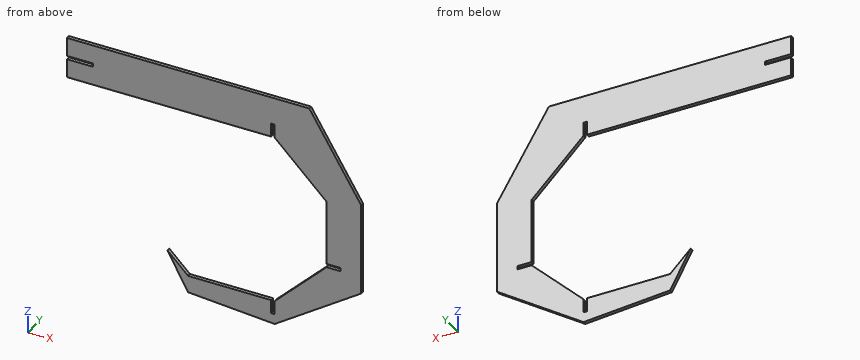
from build123d import *

# Parameters (mm, degrees)
BOSS_EXTRUDE1_DEPTH = 2.54
SKETCH2_W           = 19.05
SKETCH2_H           = 2.54
SKETCH2_W_2         = 2.54
SKETCH2_H_2         = 10.16
SKETCH2_W_3         = 10.16
CUT_EXTRUDE1_DEPTH  = 3.54


with BuildPart() as part:
    # Sketch1 → Boss-Extrude1 (new body)
    with BuildSketch(Plane(origin=(0, 0, 0), x_dir=(1, 0, 0), z_dir=(0, 1, 0))):
        Polygon((0, 0), (0, -30.48), (177.8, -30.48), (215.9, 33.02), (215.9, 101.555269233), (152.4, 144.78), (88.9, 139.7), (73.66, 111.76), (88.9, 127), (152.4, 127), (190.5, 88.9), (190.5, 38.1), (152.4, 0), align=None)
    extrude(amount=BOSS_EXTRUDE1_DEPTH)

    # Sketch2 → Cut-Extrude1 (cut, through all)
    with BuildSketch(Plane(origin=(0, 2.54, 0), x_dir=(1, 0, 0), z_dir=(0, 1, 0))):
        with Locations((9.525, -15.24)):
            Rectangle(SKETCH2_W, SKETCH2_H)
        with Locations((151.13, -5.08)):
            Rectangle(SKETCH2_W_2, SKETCH2_H_2)
        with Locations((195.58, 87.63)):
            Rectangle(SKETCH2_W_3, SKETCH2_H)
        with Locations((151.13, 132.08)):
            Rectangle(SKETCH2_W_2, SKETCH2_H_2)
    extrude(amount=-CUT_EXTRUDE1_DEPTH, mode=Mode.SUBTRACT)


solid = part.part
The listing builds one solid part. Answer for the finished solid, in the listing's coordinates (mm). Round coordinates to 2 decimals unless told otherwise and drop trailing zeros. Write each loop counter-clockwise with the first axis right and the second up, starting at its lowest first coordinate (ties: lowest second). Pieces come first, ordered by that corner, then holes. Notation, with made-up numbers: (-27.5, -11.75) - (-7.5, -11.75) arc R22 ccw to (-7.5, 27.25) - close; hole circle Ø11 at (-14, 29.25). An arc over 180 degrees is marked (long way). Use a Markdown table: item, result. Add a question column.
1. The part is cut by section A-A (y = 1.05). Write down the section's boundary in (x, z).
2. Consider line 1 (Z direction, x = 17, y = 0.6); line 2 (Z direction, x = 47.5, y = 2.45); line 3 (Z direction, x = 134, y = 2.1). Determine where each line is inside the solid, lowest interval first.
3. The part is cut by section D-D (z = -95.5). Write down the section's boundary in (x, y).
4. The part is cut by section C-C (z = -117). Write down the section's boundary in (x, y).
5. The part is cut by section B-B (x = 76.5). Write down the section's boundary in (y, z).
6. Flat-ended cylindrical pins translate along their axes: P1, Ø0.8, axis at y = 1.5, z = -87.5, coming from the -X side; P2, Ø0.8, axis at y = 1.5, z = -131.5, coming from the +X side; P3, Ø0.8, axis at x = 151, y = 1.5, coming from the -Z side. Find the tip coordinate at first contact, or state that the pin passes through.
Reported:
| question | item | result |
|---|---|---|
| 1 | outline | (0, 0) - (149.86, 0) - (149.86, 10.16) - (152.4, 10.16) - (152.4, 0) - (190.5, -38.1) - (190.5, -86.36) - (200.66, -86.36) - (200.66, -88.9) - (190.5, -88.9) - (152.4, -127) - (152.4, -137.16) - (149.86, -137.16) - (149.86, -127) - (88.9, -127) - (73.66, -111.76) - (88.9, -139.7) - (152.4, -144.78) - (215.9, -101.56) - (215.9, -33.02) - (177.8, 30.48) - (0, 30.48) - (0, 16.51) - (19.05, 16.51) - (19.05, 13.97) - (0, 13.97) - close |
| 2 | line 1 | 0 to 13.97, 16.51 to 30.48 |
| 2 | line 2 | 0 to 30.48 |
| 2 | line 3 | -143.31 to -127, 0 to 30.48 |
| 3 | outline | (183.9, 0) - (215.9, 0) - (215.9, 2.54) - (183.9, 2.54) - close |
| 4 | outline | (76.52, 0) - (78.9, 0) - (78.9, 2.54) - (76.52, 2.54) - close; (162.4, 0) - (193.21, 0) - (193.21, 2.54) - (162.4, 2.54) - close |
| 5 | outline | (0, -116.97) - (2.54, -116.97) - (2.54, -114.6) - (0, -114.6) - close; (0, 0) - (2.54, 0) - (2.54, 30.48) - (0, 30.48) - close |
| 6 | P1 | x = 200.66 |
| 6 | P2 | x = 172.5 |
| 6 | P3 | z = -144.7 |
